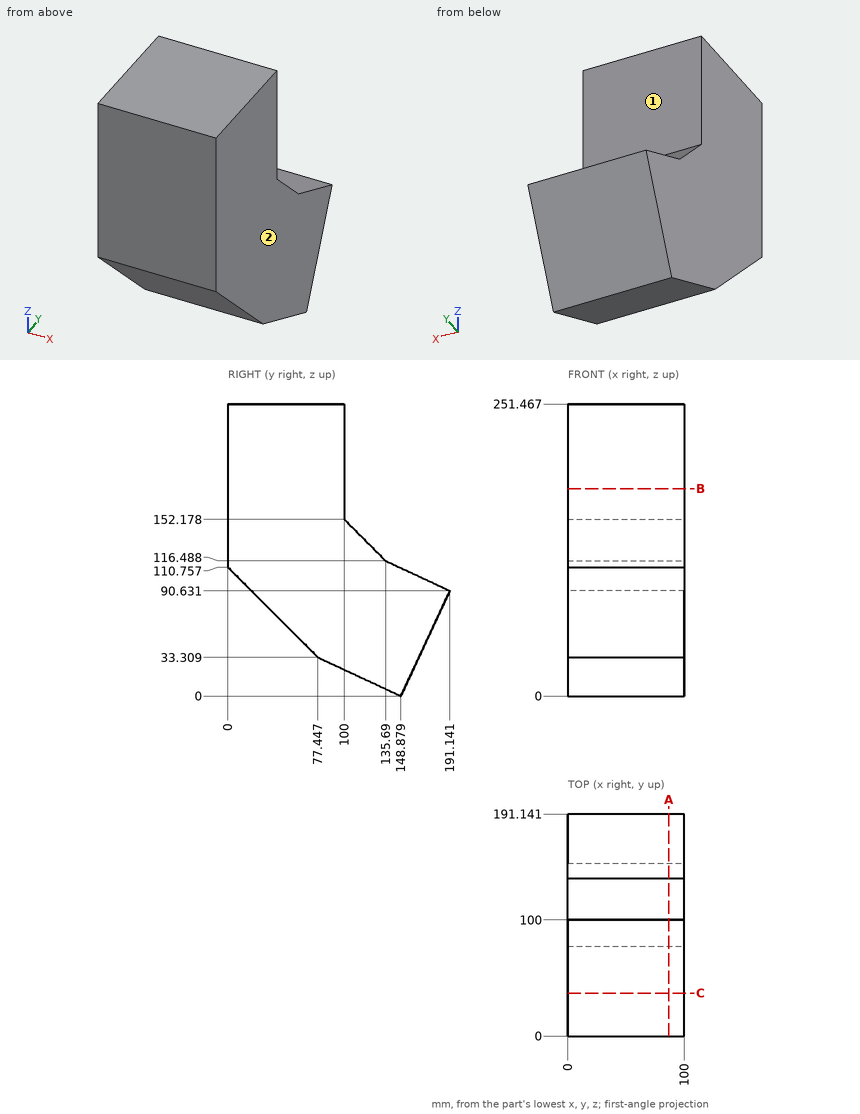
Could you check a few things on this drawing? It's one solid part, dimensions in mm from its lowest x, y, z. A direction names the side the tool comes from. Give positions to 0.01 mm unless a question says otherwise; leave off trailing zeros. Write each loop counter-clockwise with the first axis right and the second up, starting at its lowest first coordinate (ties: lowest second). Pieces come first, ordered by that corner, then holes. Notation, with made-up numbers: (12, 60.5) -> (29, 60.5) arc R16 cw to (29, 67.5) -> close; hole circle Ø6 at (-2.5, 32). An arc over 180 degrees is marked (long way). Answer as a JSON object with one key per item and string values.
Q1. Please list where these lines run through material, in increasing order: L1, parallel to Y at x = 59.5, z = 220.5; L2, parallel to Z at x = 69.5, y = 84 (1 decimal); L3, parallel to Y at x = 83, z = 46 (1 decimal).
Taken from the geometry:
{"L1": "y = 0 to 100", "L2": "z = 30.3 to 251.5", "L3": "y = 64.8 to 170.3"}
Q2. Suppose I cut it at B-B on z = 178.5. Write out the boundary of the cut face in (x, y), then the cut area to 3 significant figures.
Taken from the geometry:
{"outline": "(0, 0) -> (100, 0) -> (100, 100) -> (0, 100) -> close", "area": "10,000 mm²"}
Q3. Suppose I cut it at A-A on x = 87. Write out the boundary of the cut face in (y, z).
Taken from the geometry:
{"outline": "(0, 110.76) -> (77.45, 33.31) -> (148.88, 0) -> (191.14, 90.63) -> (135.69, 116.49) -> (100, 152.18) -> (100, 251.47) -> (0, 251.47) -> close"}
Q4. Will these pins go through, and if not, where does the flat tip stop? pin 1 Ø1.5 at (x, z) = (25, 157) entering from +Y; pin 2 Ø4 at (x, y) = (60, 171.5) entering from -Z (1 decimal); pin 3 Ø6 at (x, z) = (12.5, 47.5) entering from -Y (1 decimal).
Taken from the geometry:
{"pin 1": "stops at y = 100", "pin 2": "stops at z = 44.2", "pin 3": "stops at y = 60.3"}
Q5. Which directions (+Z, -Z, +X, -X, +Y, -Y) give clear straight access to the entire face, cutting with the end or side of a thin tool? Please do the marked faces 1 and 2.
Taken from the geometry:
{"face 1": "+Z, +X, -X, +Y", "face 2": "+Z, -Z, +X, +Y, -Y"}
Q6. Suppose I cut it at C-C on y = 37. Write out the boundary of the cut face in (x, z), then the cut area to 3 significant figures.
Taken from the geometry:
{"outline": "(0, 73.76) -> (100, 73.76) -> (100, 251.47) -> (0, 251.47) -> close", "area": "17,800 mm²"}
